```python
from build123d import *

# Parameters (mm, degrees)
F0_W     = 250
F0_H     = 27
F1_DEPTH = 7
F3_DEPTH = 25
F4_W     = 125
F4_H     = 94.8358140886
F5_DEPTH = 25


# Not quite as in the source:
# - ends of sketch curves that miss each other by under 0.0002 mm in the source are joined


with BuildPart() as f1:
    # F0 (on Top) → F1 (new body)
    with BuildSketch(Plane.XY):
        Rectangle(F0_W, F0_H)
    extrude(amount=F1_DEPTH)

    # F2 (on face) → F3 (cut)
    with BuildSketch(Plane.XY.offset(7)):
        with BuildLine():
            ThreePointArc((87, -8), (92.6568542495, -5.6568542495), (95, 0))
            ThreePointArc((95, 0), (92.6568542495, 5.6568542495), (87, 8))
            ThreePointArc((87, 8), (81.3431457505, 5.6568542495), (79, 0))
            ThreePointArc((79, 0), (81.3431457505, -5.6568542495), (87, -8))
        make_face()
        with BuildLine():
            ThreePointArc((79, 0), (81.3431457505, 5.6568542495), (87, 8))
            Line((87, 8), (71, 7.999994214))
            ThreePointArc((71, 7.999994214), (76.6568542495, 5.6568542495), (79, 0))
        make_face()
        with BuildLine():
            Line((71, -7.999994214), (87, -8))
            ThreePointArc((87, -8), (81.3431457505, -5.6568542495), (79, 0))
            ThreePointArc((79, 0), (76.6568542495, -5.6568542495), (71, -7.999994214))
        make_face()
        with BuildLine():
            ThreePointArc((71, -8), (76.6568542495, -5.6568542495), (79, 0))
            ThreePointArc((79, 0), (76.6568542495, 5.6568542495), (71, 8))
            ThreePointArc((71, 8), (63, 0), (71, -8))
        make_face()
        with BuildLine():
            ThreePointArc((-12, -8), (-6.3431457505, -5.6568542495), (-4, 0))
            ThreePointArc((-4, 0), (-6.3431457505, 5.6568542495), (-12, 8))
            ThreePointArc((-12, 8), (-20, 0), (-12, -8))
        make_face()
        with BuildLine():
            ThreePointArc((4, -8), (-1.6568542495, -5.6568542495), (-4, 0))
            ThreePointArc((-4, 0), (-6.3431457505, -5.6568542495), (-12, -8))
            Line((-12, -8), (4, -8))
        make_face()
        with BuildLine():
            ThreePointArc((-12, 8), (-6.3431457505, 5.6568542495), (-4, 0))
            ThreePointArc((-4, 0), (-1.6568542495, 5.6568542495), (4, 8))
            Line((4, 8), (-12, 8))
        make_face()
        with BuildLine():
            ThreePointArc((4, 8), (-1.6568542495, 5.6568542495), (-4, 0))
            ThreePointArc((-4, 0), (-1.6568542495, -5.6568542495), (4, -8))
            ThreePointArc((4, -8), (9.6568542495, -5.6568542495), (12, 0))
            ThreePointArc((12, 0), (9.6568542495, 5.6568542495), (4, 8))
        make_face()
        with BuildLine():
            ThreePointArc((-81.8808954364, -7.999994214), (-76.2178223077, -5.660255005), (-73.871273756, 0))
            ThreePointArc((-73.871273756, 0), (-76.2178223077, 5.660255005), (-81.8808954364, 7.999994214))
            Line((-81.8808954364, 7.999994214), (-81.8808954364, -7.999994214))
        make_face()
        with BuildLine():
            Line((-81.8808954364, -7.999994214), (-81.8808954364, 7.999994214))
            ThreePointArc((-81.8808954364, 7.999994214), (-87.531528761, 5.6534514483), (-89.871273756, 0))
            ThreePointArc((-89.871273756, 0), (-87.531528761, -5.6534514483), (-81.8808954364, -7.999994214))
        make_face()
        with BuildLine():
            ThreePointArc((-89.871273756, 0), (-87.531528761, 5.6534514483), (-81.8808954364, 7.999994214))
            Line((-81.8808954364, 7.999994214), (-97.871273756, 8))
            ThreePointArc((-97.871273756, 8), (-92.2144195065, 5.6568542495), (-89.871273756, 0))
        make_face()
        with BuildLine():
            Line((-97.32632471, -7.9814178275), (-81.8808954364, -7.999994214))
            ThreePointArc((-81.8808954364, -7.999994214), (-87.531528761, -5.6534514483), (-89.871273756, 0))
            ThreePointArc((-89.871273756, 0), (-92.0249247941, -5.4607878384), (-97.32632471, -7.9814178275))
        make_face()
        with BuildLine():
            ThreePointArc((-97.32632471, -7.9814178275), (-92.0249247941, -5.4607878384), (-89.871273756, 0))
            ThreePointArc((-89.871273756, 0), (-92.2144195065, 5.6568542495), (-97.871273756, 8))
            ThreePointArc((-97.871273756, 8), (-105.8662931823, 0.2822487793), (-98.4354198745, -7.9800839066))
            Line((-98.4354198745, -7.9800839066), (-97.32632471, -7.9814178275))
        make_face()
        with BuildLine():
            ThreePointArc((-98.4354198745, -7.9800839066), (-97.8808954364, -7.999994214), (-97.32632471, -7.9814178275))
            Line((-97.32632471, -7.9814178275), (-98.4354198745, -7.9800839066))
        make_face()
    extrude(amount=-F3_DEPTH, mode=Mode.SUBTRACT)

    # F4 (on face) → F5 (cut)
    with BuildSketch(Plane.XY.offset(7)):
        with Locations((62.5, -3.4542847425)):
            Rectangle(F4_W, F4_H)
    extrude(amount=-F5_DEPTH, mode=Mode.SUBTRACT)


solid = f1.part
```
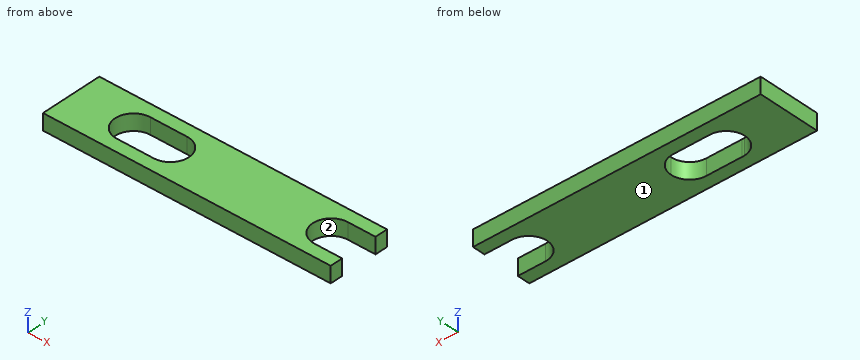
Here's how the part is built. I have some questions about the finished solid (model axes, mm). Face numbers are marked on the shaded views. Coordinates: 2 decimals unless noted, no trailing zeros. Loops run counter-clockwise (first coordinate to the right, second up) from the corner with the lowest first, then second, coordinate; pieces in that order, holes last. Notation, with made-up numbers: (22.5, 60.25) - (78.5, 60.25) arc R20 ccw to (78.5, 65.25) - close; hole circle Ø5 at (0.5, 64.5). An arc over 180 degrees is marked (long way). Return JSON: item names as keys, results as strings. Group by question number.
Item 1: If we section it at A-A on y = 4.25: Write out the boundary of the cut face in (x, z).
Item 2: Will these pins go through, and if not, where does the flat tip stop? P1, Ø1.5, axis at x = -104, y = -5, coming from the -Z side; P2, Ø1, axis at y = -6, z = 5.5, coming from the +X side.
Item 3: I need wall thicknesses on line 1 (X direction, y = -0.5, z = 3.5); line 2 (Y direction, x = -92, z = 5.25); line 3 (Y direction, x = -80.5, z = 6.25). Which ranges of each line are inside material? Lowest first, please. Write a range as from..to.
Item 4: We'd pull the mould along Y, two halves only. Please class the marked faces 1 and 2: +Y half, -Y half, draft (parallel to the pull), parting line (faces both ways), or undercut.
Calculated:
{
 "1": {"outline": "(-125, 0) - (-104.65, 0) - (-104.65, 7) - (-125, 7) - close; (-75.09, 0) - (-18.78, 0) - (-18.78, 7) - (-75.09, 7) - close"},
 "2": {"P1": "stops at z = 0", "P2": "stops at x = -16.66"},
 "3": {"line 1": "x = -125..-105.86, -73.89..-19.98", "line 2": "y = -13.5..-7.99, 8..13.5", "line 3": "y = -13.5..-7.88, 7.88..13.5"},
 "4": {"face 1": "draft", "face 2": "undercut"}
}
